Could you check a few things on this model? Use its own coordinates, in mm. A direction names the side the tool comes from. Give positions to 0.01 mm unless a question says otherwise; leave off trailing zeros. Write each loop counter-clockwise with the first axis right and the second up, starting at its lowest first coordinate (ties: lowest second). Pieces come first, ordered by that corner, then holes. Notation, with made-up numbers: (79, 48) -> (118, 48) arc R28 ccw to (118, 71) -> close; hole circle Ø2 at (9, 84). An arc over 180 degrees is marked (long way). One line per question, with ' | ' between items.
from build123d import *

# Parameters (mm, degrees)
SKETCH2_R               = 4.365625
SKETCH2_R_2             = 1.5875
CUT_EXTRUDE1_DEPTH      = 1
CUT_EXTRUDE1_DEPTH_BACK = 7.35
SKETCH3_R               = 3.96875
CUT_EXTRUDE2_DEPTH      = 3.175


with BuildPart() as part:
    # Sketch1 → Revolve1 (revolve)
    with BuildSketch(Plane.XY):
        Polygon((0, 0), (-27, 0), (-27, 3.175), (-25.4, 3.175), (-25.4, 6.35), (0, 6.35), align=None)
    revolve(axis=Axis((0, 6.35, 0), (0, -1, 0)))

    # Sketch2 → Cut-Extrude1 (cut, two sides)
    with BuildSketch(Plane(origin=(0, 6.35, 0), x_dir=(1, 0, 0), z_dir=(0, 1, 0))) as cut_extrude1_sk:
        Circle(SKETCH2_R)
        with Locations((12.7, 0)):
            Circle(SKETCH2_R_2)
    extrude(amount=CUT_EXTRUDE1_DEPTH, mode=Mode.SUBTRACT)
    extrude(cut_extrude1_sk.sketch, amount=-CUT_EXTRUDE1_DEPTH_BACK, mode=Mode.SUBTRACT)

    # Sketch3 → Cut-Extrude2 (cut)
    with BuildSketch(Plane.XZ):
        with Locations((0, 12.7)):
            Circle(SKETCH3_R)
    extrude(amount=-CUT_EXTRUDE2_DEPTH, mode=Mode.SUBTRACT)


solid = part.part
Q1. Will these pins go through, and if not, where does the flat tip stop? pin 1 (6.5 mm diameter, centred on x = 0, z = 12.5, fed in from -Y) (3 decimals); pin 2 (1.5 mm diameter, centred on x = 9, y = 3, fed in from -Z).
Answer below:
pin 1: stops at y = 3.175 | pin 2: stops at z = -25.71
Q2. Imagine slicing it at B-B on x = 0. Please give me the cut outline in (y, z) (3 decimals).
Answer below:
outline: (0, -27) -> (3.175, -27) -> (3.175, -25.4) -> (6.35, -25.4) -> (6.35, -4.366) -> (0, -4.366) -> close; (0, 4.366) -> (6.35, 4.366) -> (6.35, 25.4) -> (3.175, 25.4) -> (3.175, 27) -> (0, 27) -> (0, 16.669) -> (3.175, 16.669) -> (3.175, 8.731) -> (0, 8.731) -> close
Q3. On a 3-axis mill with a long thin cutter (end or side, diameter ignored), from which of +Z, -Z, +X, -X, +Y, -Y can I reach the whole of each face in a straight line? I mean faces 4 (the cylindrical face through (5.506, 4.785, 24.796)), 5 (the flat face through (0, 3.175, 13)), 6 (the cylindrical face through (-3.46, 3.22, 2.66)). Say none if no direction works.
Answer below:
face 4: +Y | face 5: -Y | face 6: +Y, -Y
Q4. Imagine slicing it at D-D on x = -8. Please give me the cut outline in (y, z) (3 decimals), and give its area (3 significant figures).
Answer below:
outline: (0, -25.788) -> (3.175, -25.788) -> (3.175, -24.107) -> (6.35, -24.107) -> (6.35, 24.107) -> (3.175, 24.107) -> (3.175, 25.788) -> (0, 25.788) -> close | area: 317 mm^2
Q5. If I drill on line 1 along X through (y, z) = (4.5, 0); line 2 along X through (y, z) = (2.5, 0); line 3 along Z through (x, y) = (0, 3.75), over which ranges is the centre line in solid material (lowest first)?
Answer below:
line 1: x = -25.4 to -4.37, 4.37 to 11.11, 14.29 to 25.4 | line 2: x = -27 to -4.37, 4.37 to 11.11, 14.29 to 27 | line 3: z = -25.4 to -4.37, 4.37 to 25.4
Q6. Imagine slicing it at A-A on z = 0. Count the separate pieces of the cut face and the enclosed holes in it, and give its area (3 significant figures).
Answer below:
separate pieces: 3 | enclosed holes: 0 | area: 257 mm^2
Q7. If we mould it in two halves opening along X, with no side actions, what happens to faces 1 (the flat face through (-5, 6.35, 0)), 2 (the cylindrical face through (-0.86, 1.565, 8.826)), 3 (the cylindrical face through (5.85, 1.61, 26.36))? For each: +X half, -X half, draft (parallel to the pull), parting line (faces both ways), or undercut.
Answer below:
face 1: draft | face 2: undercut | face 3: parting line
Q8. Imagine slicing it at C-C on z = -18. Please give me the cut outline in (x, y) (3 decimals), and give its area (3 significant figures).
Answer below:
outline: (-20.125, 0) -> (20.125, 0) -> (20.125, 3.175) -> (17.921, 3.175) -> (17.921, 6.35) -> (-17.921, 6.35) -> (-17.921, 3.175) -> (-20.125, 3.175) -> close | area: 242 mm^2
